Can you work these out from the drawing? Everything is in mm from the part's minimum corner. Round coordinates to 2 decimals unless told otherwise and drop trailing zeros. Order: outer loops, then holes, each group sorted by start corner. A loop starts at its lowest first (then second) coordinate and runs counter-clockwise, first axis right, second up. Notation, with made-up numbers: M -22,21 L 23,21 A10 ccw 23,32 Z; hole C 10,82.25 d10. An arc over 180 degrees is marked long. Write each question's results on one line, items separated by ' | '. Start each with the question number.
1. Please list where these lines run through material, in increasing order: L1, parallel to Z at x = 98, y = 3.4; L2, parallel to X at y = 3.75, z = 19.5; L3, parallel to X at y = 4.45, z = 21.5.
2. Suppose I cut it at A-A on x = 58. Write out the boundary of the cut face in (y, z), and give its area (4 significant figures).
3. Suppose I cut it at B-B on y = 4.15. Write out the boundary of the cut face in (x, z), and give its area (3 significant figures).
4. I'm going to push a flat-ended pin straight in: pin 1 (5.5 mm diameter, centred on x = 138, z = 18, fed in from +Y). Where does the tip first touch, or does it pass through?
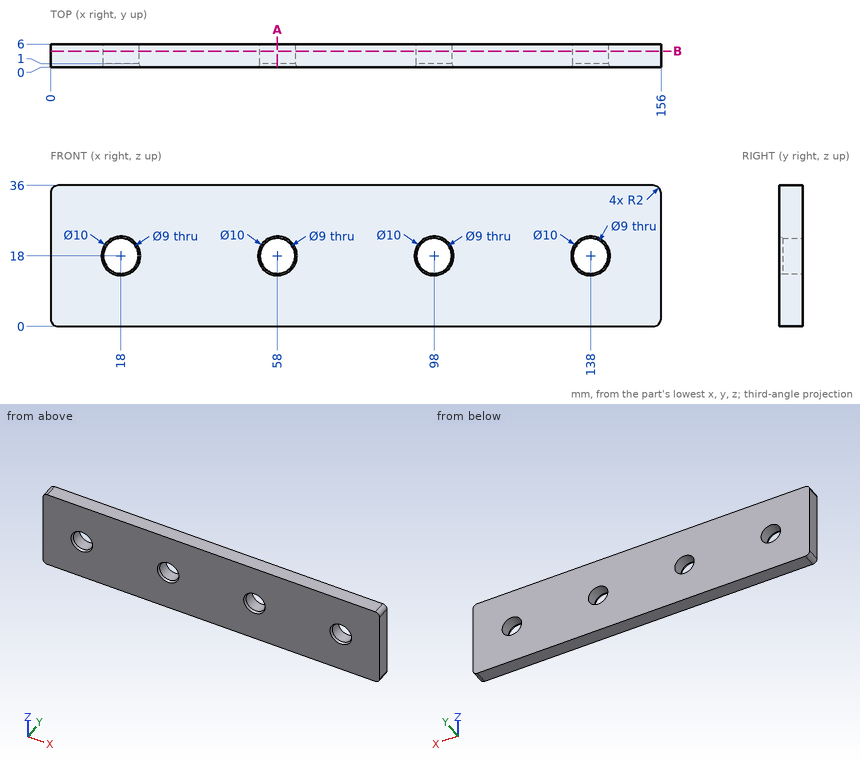
Filled sheet:
1) L1: z = 0 to 13.5, 22.5 to 36 | L2: x = 0 to 13.76, 22.24 to 53.76, 62.24 to 93.76, 102.24 to 133.76, 142.24 to 156 | L3: x = 0 to 15.17, 20.83 to 55.17, 60.83 to 95.17, 100.83 to 135.17, 140.83 to 156
2) outline: M 0,0 L 6,0 L 6,13.5 L 1,13.5 L 0,13 Z; M 0,23 L 1,22.5 L 6,22.5 L 6,36 L 0,36 Z | area: 161.5 mm^2
3) outline: M 0,2 A2 ccw 2,0 L 154,0 A2 ccw 156,2 L 156,34 A2 ccw 154,36 L 2,36 A2 ccw 0,34 Z; hole C 18,18 d9; hole C 58,18 d9; hole C 98,18 d9; hole C 138,18 d9 | area: 5,360 mm^2
4) pin 1: passes through
